Source: CAD feature listing. Evaluate the final solid. Frame: model axes, mm. Give positions to 0.01 mm unless a question says otherwise; leave off trailing zeros. Write each loop counter-clockwise with the first axis right and the second up, starting at its lowest first coordinate (ties: lowest second). Pieces come first, ordered by that corner, then holes. Notation, with made-up numbers: (12, 15) -> (42, 15) arc R18 ccw to (42, 19) -> close; hole circle Ø10 at (62.5, -15.5). An arc over 180 degrees is marked (long way). Write item = value, one per line.
from build123d import *

# Parameters (mm, degrees)
SKETCH1_R           = 158.75
BOSS_EXTRUDE1_DEPTH = 28.575


with BuildPart() as part:
    # Sketch1 → Boss-Extrude1 (new, symmetric)
    with BuildSketch(Plane(origin=(0, 0, 0), x_dir=(0, 1, 0), z_dir=(0, 0, 1))):
        with Locations(Location((0, 0, 0), (0, 0, 270))):
            Circle(SKETCH1_R)
        with BuildLine():
            Line((21.800803257, 109.978472222), (13.669356496, 68.957777656))
            ThreePointArc((13.669356496, 68.957777656), (14.983750202, 60.395804017), (21.482165761, 54.668185085))
            ThreePointArc((21.482165761, 54.668185085), (29.36875, 50.868167155), (36.602954182, 45.93819382))
            ThreePointArc((36.602954182, 45.93819382), (44.81242546, 43.174210327), (52.88450899, 46.316898807))
            Line((52.88450899, 46.316898807), (84.343749185, 73.869285555))
            ThreePointArc((84.343749185, 73.869285555), (118.234118252, 68.2625), (106.144552443, 36.109186667))
            Line((106.144552443, 36.109186667), (66.553865487, 22.640878849))
            ThreePointArc((66.553865487, 22.640878849), (59.796175661, 17.22159369), (58.085119943, 8.729991265))
            ThreePointArc((58.085119943, 8.729991265), (58.7375, 0), (58.085119943, -8.729991265))
            ThreePointArc((58.085119943, -8.729991265), (59.796175661, -17.22159369), (66.553865487, -22.640878849))
            Line((66.553865487, -22.640878849), (106.144552443, -36.109186667))
            ThreePointArc((106.144552443, -36.109186667), (118.234118252, -68.2625), (84.343749185, -73.869285555))
            Line((84.343749185, -73.869285555), (52.88450899, -46.316898807))
            ThreePointArc((52.88450899, -46.316898807), (44.81242546, -43.174210327), (36.602954182, -45.93819382))
            ThreePointArc((36.602954182, -45.93819382), (29.36875, -50.868167155), (21.482165761, -54.668185085))
            ThreePointArc((21.482165761, -54.668185085), (14.983750202, -60.395804017), (13.669356496, -68.957777656))
            Line((13.669356496, -68.957777656), (21.800803257, -109.978472222))
            ThreePointArc((21.800803257, -109.978472222), (0, -136.525), (-21.800803257, -109.978472222))
            Line((-21.800803257, -109.978472222), (-13.669356496, -68.957777656))
            ThreePointArc((-13.669356496, -68.957777656), (-14.983750202, -60.395804017), (-21.482165761, -54.668185085))
            ThreePointArc((-21.482165761, -54.668185085), (-29.36875, -50.868167155), (-36.602954182, -45.93819382))
            ThreePointArc((-36.602954182, -45.93819382), (-44.81242546, -43.174210327), (-52.88450899, -46.316898807))
            Line((-52.88450899, -46.316898807), (-84.343749185, -73.869285555))
            ThreePointArc((-84.343749185, -73.869285555), (-118.234118252, -68.2625), (-106.144552443, -36.109186667))
            Line((-106.144552443, -36.109186667), (-66.553865487, -22.640878849))
            ThreePointArc((-66.553865487, -22.640878849), (-59.796175661, -17.22159369), (-58.085119943, -8.729991265))
            ThreePointArc((-58.085119943, -8.729991265), (-58.7375, 0), (-58.085119943, 8.729991265))
            ThreePointArc((-58.085119943, 8.729991265), (-59.796175661, 17.22159369), (-66.553865487, 22.640878849))
            Line((-66.553865487, 22.640878849), (-106.144552443, 36.109186667))
            ThreePointArc((-106.144552443, 36.109186667), (-118.234118252, 68.2625), (-84.343749185, 73.869285555))
            Line((-84.343749185, 73.869285555), (-52.88450899, 46.316898807))
            ThreePointArc((-52.88450899, 46.316898807), (-44.81242546, 43.174210327), (-36.602954182, 45.93819382))
            ThreePointArc((-36.602954182, 45.93819382), (-29.36875, 50.868167155), (-21.482165761, 54.668185085))
            ThreePointArc((-21.482165761, 54.668185085), (-14.983750202, 60.395804017), (-13.669356496, 68.957777656))
            Line((-13.669356496, 68.957777656), (-21.800803257, 109.978472222))
            ThreePointArc((-21.800803257, 109.978472222), (0, 136.525), (21.800803257, 109.978472222))
        make_face(mode=Mode.SUBTRACT)
    extrude(amount=BOSS_EXTRUDE1_DEPTH, both=True)


solid = part.part
1) Draft query along X for faces 1 (the cylindrical face through (151.42, 47.68, 0.4)), 2 (the cylindrical face through (-67.783, -118.503, 0.4)). Return one class per face: pulls with the +X half, pulls with the -X half, needs draft (parallel to the pull), parting line crosses it, or undercut.
Computed:
face_1 = parting line crosses it
face_2 = undercut
2) Cut plane C-C (y = 111.5). Return the cut outline in (x, z) (3 decimals), then the cut area to 3 significant figures.
Computed:
outline = (-113.001, -28.575) -> (-75.518, -28.575) -> (-75.518, 28.575) -> (-113.001, 28.575) -> close; (-38.782, -28.575) -> (38.782, -28.575) -> (38.782, 28.575) -> (-38.782, 28.575) -> close; (75.518, -28.575) -> (113.001, -28.575) -> (113.001, 28.575) -> (75.518, 28.575) -> close
area = 8,720 mm²
3) Cut plane D-D (x = 63). Return the cut outline in (y, z) (3 decimals).
Computed:
outline = (-145.714, -28.575) -> (-120.428, -28.575) -> (-120.428, 28.575) -> (-145.714, 28.575) -> close; (-71.933, -28.575) -> (-13.915, -28.575) -> (-13.915, 28.575) -> (-71.933, 28.575) -> close; (13.915, -28.575) -> (71.933, -28.575) -> (71.933, 28.575) -> (13.915, 28.575) -> close; (120.428, -28.575) -> (145.714, -28.575) -> (145.714, 28.575) -> (120.428, 28.575) -> close
4) Cut plane A-A (y = 0). Return the cut outline in (x, z) (3 decimals).
Computed:
outline = (-158.75, -28.575) -> (-136.525, -28.575) -> (-136.525, 28.575) -> (-158.75, 28.575) -> close; (136.525, -28.575) -> (158.75, -28.575) -> (158.75, 28.575) -> (136.525, 28.575) -> close
5) Material intervals for L1, parallel to X at y = 64, z = 5.5; L2, parallel to X at y = 118, z = 10.5; L3, parallel to Y at x = 57.15, z = -15.5, sorted ascending.
Computed:
L1 = -145.28 to -56.05, -21.44 to 21.44, 56.05 to 145.28
L2 = -106.2 to -68.66, -45.64 to 45.64, 68.66 to 106.2
L3 = -148.11 to -121.21, -65.25 to -17.52, 17.52 to 65.25, 121.21 to 148.11
6) Contact query for flat-ended pins moving along their axis: pin 1 (2 mm diameter, centred on y = 114, z = 2, fed in from -X); pin 2 (12 mm diameter, centred on x = -68.5, y = 3.5, fed in from -Z); pin 3 (8 mm diameter, centred on y = 77, z = -3, fed in from +X); pin 4 (5 mm diameter, centred on y = 115, z = -20, fed in from -X). Output: stop coordinate, or through.
Computed:
pin_1 = -111.5
pin_2 = through
pin_3 = 140.97
pin_4 = -112.01
